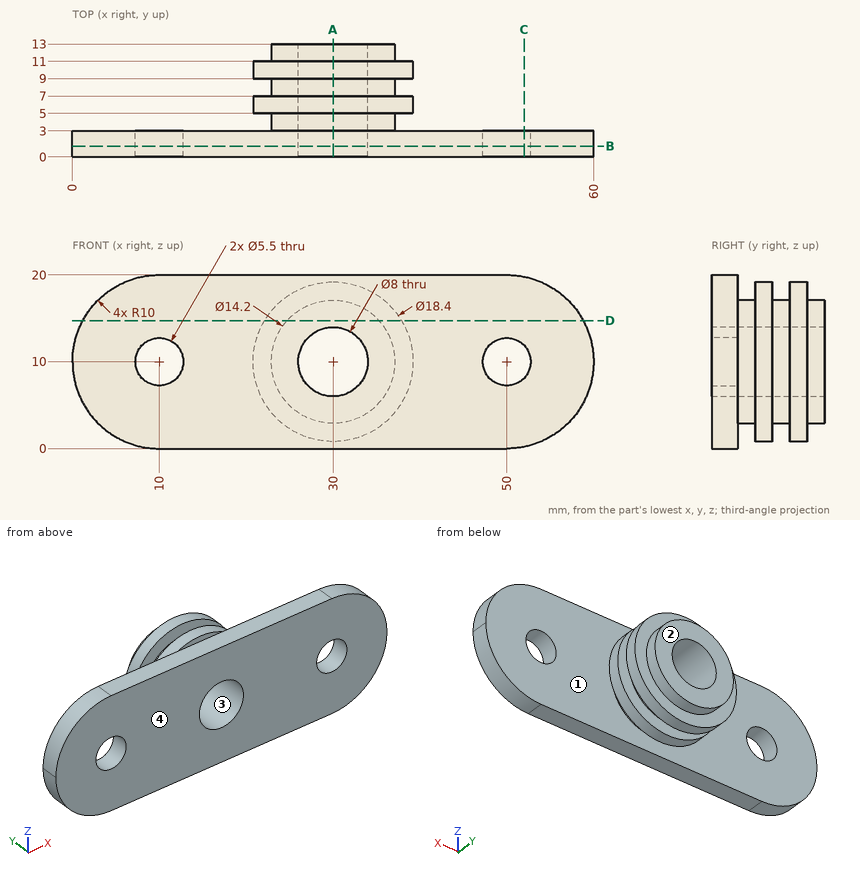
Geometry: see drawing. Coordinates: mm, zero at the bounding-box minimum. A direction names the side the tool comes from. Round coordinates to 2 decimals unless told otherwise and drop trailing zeros. Write each loop counter-clockwise with the first axis right and the second up, starting at its lowest first coordinate (ties: lowest second). Pieces come first, ordered by that corner, then holes.
1) Cut plane B-B (y = 1.25). Count the separate pieces of the cut face and the enclosed holes in it, then the cut area to 3 significant figures.
2) Draft query along X for the marked faces 3 and 4. Return one class per face: pulls with the +X half, pulls with the -X half, needs draft (parallel to the pull), parting line crosses it, or undercut.
3) Contact query for flat-ended pins moving along their axis: P1, Ø5, axis at x = 11, z = 5.5, coming from the +Y side; P2, Ø7, axis at x = 30, z = 10, coming from the -Y side; P3, Ø5, axis at y = 9.5, z = 11.5, coming from the -X side. Output: stop coordinate, or through.
4) Cut plane D-D (z = 14.75). Return the cut outline in (x, y), then the cut area to 3 significant figures.
5) Ray query, L1, parallel to Y at x = 38, z = 12; L2, parallel to X at y = 2.3, z = 10; L3, parallel to Y at x = 19, z = 18. Return the intervals inside material, ascending.
6) Cut plane A-A (x = 30). Return the cut outline in (y, z).
7) Cut plane C-C (x = 52). Return the cut outline in (y, z).
8) Reachability of the marked faces 1 and 2 from +Z, -Z, +X, -X, +Y, -Y: full face, straight path, thin tool, end or side. Return the list, or none.
Geometry says:
1. separate pieces: 1
1. enclosed holes: 3
1. area: 1,020 mm2
2. face 3: undercut
2. face 4: needs draft
3. P1: stops at y = 3
3. P2: passes through
3. P3: stops at x = 20.8
4. outline: (1.2, 0) - (58.8, 0) - (58.8, 3) - (35.28, 3) - (35.28, 5) - (37.88, 5) - (37.88, 7) - (35.28, 7) - (35.28, 9) - (37.88, 9) - (37.88, 11) - (35.28, 11) - (35.28, 13) - (24.72, 13) - (24.72, 11) - (22.12, 11) - (22.12, 9) - (24.72, 9) - (24.72, 7) - (22.12, 7) - (22.12, 5) - (24.72, 5) - (24.72, 3) - (1.2, 3) - close
4. area: 299 mm2
5. L1: y = 0 to 3, 5 to 7, 9 to 11
5. L2: x = 0 to 7.25, 12.75 to 26, 34 to 47.25, 52.75 to 60
5. L3: y = 0 to 3
6. outline: (0, 0) - (3, 0) - (3, 2.9) - (5, 2.9) - (5, 0.8) - (7, 0.8) - (7, 2.9) - (9, 2.9) - (9, 0.8) - (11, 0.8) - (11, 2.9) - (13, 2.9) - (13, 6) - (0, 6) - close; (0, 14) - (13, 14) - (13, 17.1) - (11, 17.1) - (11, 19.2) - (9, 19.2) - (9, 17.1) - (7, 17.1) - (7, 19.2) - (5, 19.2) - (5, 17.1) - (3, 17.1) - (3, 20) - (0, 20) - close
7. outline: (0, 0.2) - (3, 0.2) - (3, 8.11) - (0, 8.11) - close; (0, 11.89) - (3, 11.89) - (3, 19.8) - (0, 19.8) - close
8. face 1: none
8. face 2: +Z, -Z, +X, -X, +Y
